Input: dimensioned drawing with shaded views. Units: mm. Origin: part minimum x, y, z. A direction names the side the tool comes from. Give positions to 0.01 mm unless a question says otherwise; leave off trailing zeros. Write each loop counter-clockwise with the first axis right and the second up, starting at its lowest first coordinate (ties: lowest second). Pieces come first, ordered by that corner, then holes. Notation, with made-up numbers: (-19, 50.5) -> (1, 50.5) arc R16 cw to (1, 75.5) -> close; hole circle Ø4 at (53, 80.25). An arc over 180 degrees is marked (long way). Answer as a JSON object with one key per item and string values.
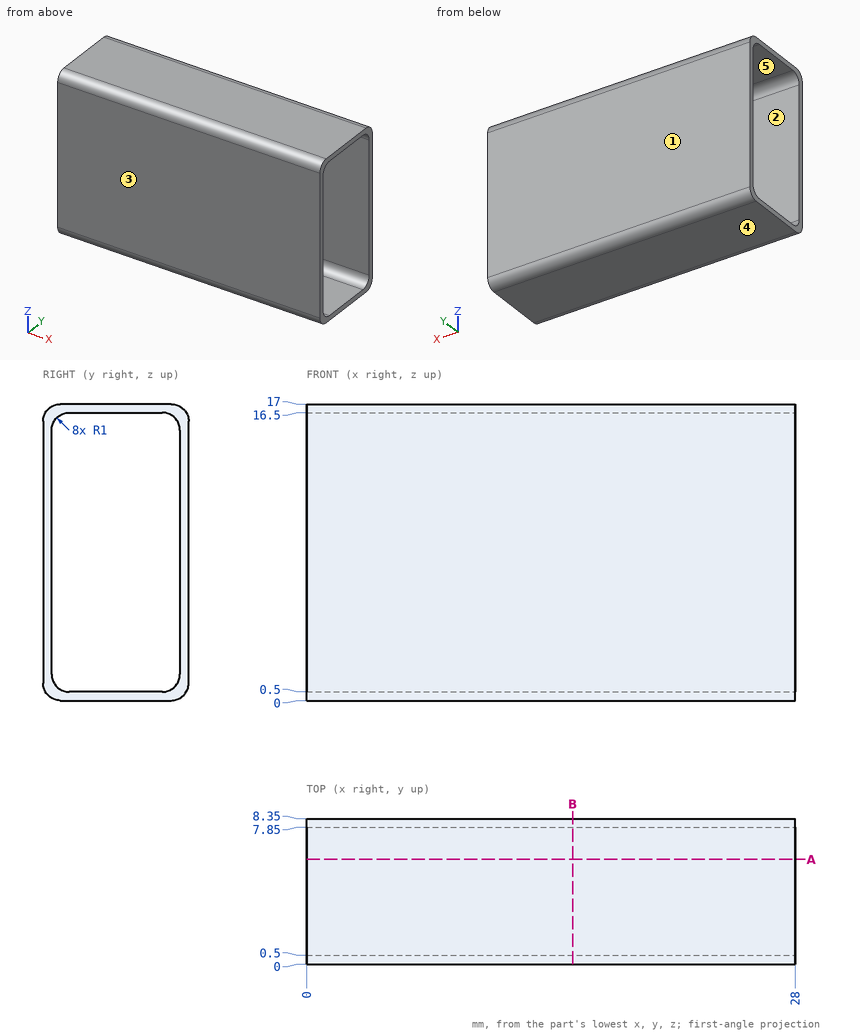
Q1. Material intervals for L1, parallel to Y at x = 11, z = 2; L2, parallel to Z at x = 25.5, y = 1.5; L3, parallel to Z at x = 17.5, y = 7.25, sorted ascending. Write a range as from..to.
Values:
{"L1": "0..0.5, 7.85..8.35", "L2": "0..0.5, 16.5..17", "L3": "0..0.58, 16.42..17"}
Q2. Mould query, pull axis Z, two halves, no side actions, for the marked faces 3, 4 and 5. Classes: pulls with the +Z half, pulls with the -Z half, needs draft (parallel to the pull), parting line crosses it, or undercut.
Values:
{"face 3": "needs draft", "face 4": "pulls with the -Z half", "face 5": "undercut"}
Q3. Cut plane B-B (x = 15.25). Return the cut outline in (y, z).
Values:
{"outline": "(0, 1) arc R1 ccw to (1, 0) -> (7.35, 0) arc R1 ccw to (8.35, 1) -> (8.35, 16) arc R1 ccw to (7.35, 17) -> (1, 17) arc R1 ccw to (0, 16) -> close; hole (0.5, 1.5) arc R1 ccw to (1.5, 0.5) -> (6.85, 0.5) arc R1 ccw to (7.85, 1.5) -> (7.85, 15.5) arc R1 ccw to (6.85, 16.5) -> (1.5, 16.5) arc R1 ccw to (0.5, 15.5) -> close"}
Q4. Set-up query: the marked faces 1 and 2. Return all of +Z, -Z, +X, -X, +Y, -Y with unobstructed straight access to the full face (end or side cutting, diameter ignored); none if empty.
Values:
{"face 1": "+Z, -Z, +X, -X, +Y", "face 2": "+X, -X"}
Q5. First-contact query: P1, Ø2, axis at x = 15.5, y = 2.5, coming from the -Z side. Flat tip, straight axial feed; report the tip coordinate or a pass-through.
Values:
{"P1": "z = 0"}
Q6. Cut plane A-A (y = 6). Return the cut outline in (x, z), and give its area (3 significant figures).
Values:
{"outline": "(0, 0) -> (28, 0) -> (28, 0.5) -> (0, 0.5) -> close; (0, 16.5) -> (28, 16.5) -> (28, 17) -> (0, 17) -> close", "area": "28.0 mm²"}
